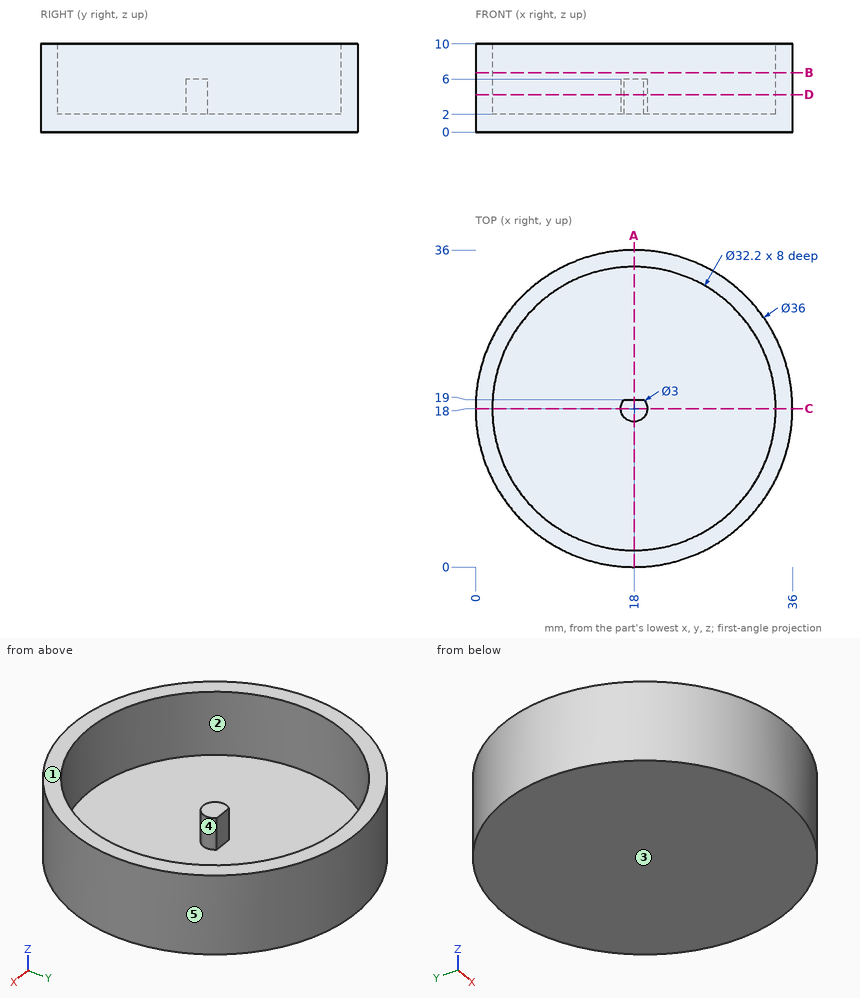
Geometry check sheet. Reference: drawing and pictorial views, mm from the part's lowest x, y, z. A direction names the side the tool comes from. Round coordinates to 2 decimals unless told otherwise and drop trailing zeros. Loops run counter-clockwise (first coordinate to the right, second up) from the corner with the lowest first, then second, coordinate; pieces in that order, holes last. Notation, with made-up numbers: (-31, 19.5) - (21, 19.5) arc R18 ccw to (21, 47.5) - close; hole circle Ø9 at (-11, -0.75). An arc over 180 degrees is marked (long way). Use a Markdown table: item, result.
Q1. Cross-section at D-D on z = 4.25. Record the cut outline in (x, y).
Solutions:
| item | result |
|---|---|
| outline | circle Ø36 at (18, 18); (16.88, 19) arc R1.5 ccw (long way) to (19.12, 19) - close; hole circle Ø32.2 at (18, 18) |
Q2. Draft check along Y on the marked faces 3, 4 and 5. Enter one of: released by +Y, released by -Y, zero draft, split by the parting line, or undercut.
Solutions:
| item | result |
|---|---|
| face 3 | zero draft |
| face 4 | undercut |
| face 5 | split by the parting line |
Q3. Material ranges on line 1 (Y direction, x = 18, z = 5.5); line 2 (Y direction, x = 18, z = 7.25); line 3 (Z direction, x = 10.5, y = 24), recorded low to high.
Solutions:
| item | result |
|---|---|
| line 1 | y = 0 to 1.9, 16.5 to 19, 34.1 to 36 |
| line 2 | y = 0 to 1.9, 34.1 to 36 |
| line 3 | z = 0 to 2 |
Q4. Cross-section at B-B on z = 6.75. Record the cut outline in (x, y), plus the area to 3 significant figures.
Solutions:
| item | result |
|---|---|
| outline | circle Ø36 at (18, 18); hole circle Ø32.2 at (18, 18) |
| area | 204 mm2 |
Q5. Cross-section at C-C on y = 18. Record the cut outline in (x, z).
Solutions:
| item | result |
|---|---|
| outline | (0, 0) - (36, 0) - (36, 10) - (34.1, 10) - (34.1, 2) - (19.5, 2) - (19.5, 6) - (16.5, 6) - (16.5, 2) - (1.9, 2) - (1.9, 10) - (0, 10) - close |
Q6. Go/stop test with flat-tipped pins: P1, Ø1.1, axis at x = 18.5, z = 5, coming from the +Y side; P2, Ø5, axis at x = 23.5, z = 4.5, coming from the -Y side; P3, Ø5, axis at y = 26, z = 8, coming from the -X side. Record where each tip stops, or that it passes through.
Solutions:
| item | result |
|---|---|
| P1 | stops at y = 36 |
| P2 | stops at y = 0.25 |
| P3 | stops at x = 0.86 |
Q7. Cross-section at A-A on x = 18. Record the cut outline in (y, z).
Solutions:
| item | result |
|---|---|
| outline | (0, 0) - (36, 0) - (36, 10) - (34.1, 10) - (34.1, 2) - (19, 2) - (19, 6) - (16.5, 6) - (16.5, 2) - (1.9, 2) - (1.9, 10) - (0, 10) - close |
Q8. Access from +Z, -Z, +X, -X, +Y, -Y to the whole of each face (thin tool, end or side, straight path). Record for the marked faces 1 and 2.
Solutions:
| item | result |
|---|---|
| face 1 | +Z, +X, -X, +Y, -Y |
| face 2 | +Z |
